Autodesk Inventor part; units mm, degrees
ref_plane "Start plane" through (0, 0, 0) normal (0, 0, 1) x (1, 0, 0)
ref_plane "End plane" through (0, 0, 609.6) normal (0, 0, 1) x (1, 0, 0)
ref_plane "YZ Plane" through (0, 0, 0) normal (1, 0, 0) x (0, 1, 0)
ref_plane "Start plane" through (0, 0, 0) normal (0, 0, 1) x (1, 0, 0)
ref_plane "End plane" through (0, 0, 609.6) normal (0, 0, 1) x (1, 0, 0)
sketch "Sketch" plane through (0, 0, 0) normal (0, 0, 1) x (1, 0, 0)
  line L0 (-25.4, -12.7) -> (-25.4, 12.7)
  line L1 (-12.7, 25.4) -> (12.7, 25.4)
  line L2 (25.4, 12.7) -> (25.4, -12.7)
  line L3 (12.7, -25.4) -> (-12.7, -25.4)
  arc A0 (-25.4, -12.7) -> (-12.7, -25.4) centre (-12.7, -12.7) ccw
  arc A1 (-12.7, 25.4) -> (-25.4, 12.7) centre (-12.7, 12.7) ccw
  arc A2 (25.4, 12.7) -> (12.7, 25.4) centre (12.7, 12.7) ccw
  arc A3 (12.7, -25.4) -> (25.4, -12.7) centre (12.7, -12.7) ccw
  arc A4 (-12.7, 19.05) -> (-19.05, 12.7) centre (-12.7, 12.7) ccw
  line L4 (-12.7, 19.05) -> (12.7, 19.05)
  arc A5 (19.05, 12.7) -> (12.7, 19.05) centre (12.7, 12.7) ccw
  line L5 (19.05, 12.7) -> (19.05, -12.7)
  arc A6 (12.7, -19.05) -> (19.05, -12.7) centre (12.7, -12.7) ccw
  line L6 (12.7, -19.05) -> (-12.7, -19.05)
  arc A7 (-19.05, -12.7) -> (-12.7, -19.05) centre (-12.7, -12.7) ccw
  line L7 (-19.05, -12.7) -> (-19.05, 12.7)
  line L8 (0, 39.2424) -> (0, -39.2424) construction
  line L9 (-39.2424, 0) -> (39.2424, 0) construction
  dimension "d10" = 50.8
  dimension "d11" = 50.8
  dimension "d12" = 6.35
  dimension "d15" = 25.4
  dimension "d16" = 25.4
  dimension "d17" = 12.7
extrude "Body" add sketch "Sketch" along normal up to surface (609.6 mm away) from surface at 0
sketch "Sketch3" plane through (0, 0, 0) normal (0, 0, 1) x (1, 0, 0)
  line L0 (0, 0) -> (10, 0)
ref_plane "Work Plane3" through (0, 0, 0) normal (0, -1, 0) x (1, 0, 0)
sketch "Sketch4" plane through (0, 0, 0) normal (0, -1, 0) x (1, 0, 0)
  line L0 (-2, 0) -> (12, 0)
  line L1 (-2, 609.6) -> (12, 609.6)
  dimension "d19" = 609.6
sketch "Sketch5" plane through (25.4, -12.7, 609.6) normal (1, 0, 0) x (0, 0, -1)
  line L0 (609.6, 25.4) -> (609.6, 38.1)
  line L1 (609.6, 25.4) -> (609.6, 0)
  line L2 (609.6, -12.7) -> (609.6, 0)
  line L3 (609.6, 38.1) -> (606.895, 38.1)
  line L4 (606.895, 38.1) -> (609.5275, 8.0103)
  line L5 (609.6, -12.7) -> (590.55, -12.7)
  arc A0 (609.6, 6.35) -> (609.5275, 8.0103) centre (590.55, 6.35) ccw
  arc A1 (590.55, -12.7) -> (609.6, 6.35) centre (590.55, 6.35) ccw
  line L6 (0, 25.4) -> (0, 38.1)
  line L7 (0, 25.4) -> (0, 0)
  line L8 (0, -12.7) -> (0, 0)
  line L9 (0, -12.7) -> (4.4444, -12.7)
  line L10 (4.4444, -12.7) -> (0, 38.1)
  point P0 (609.6, 12.7)
  dimension "d20" = 5
  dimension "d23" = 19.05
extrude "Extrusion2" cut sketch "Sketch5" against normal through all
hole "Hole1" at (25.4, -6.35, 19.05) direction (-1, 0, 0) diameter 12.7 end through all
sketch "Sketch6" plane through (25.4, 12.7, 608.4889) normal (1, 0, 0) x (0, 0, -1)
  point P0 (608.4889, -12.7)
  point P1 (557.6889, -6.35)
  dimension "d33" = 50.8
  dimension "d34" = 6.35
hole "Hole2" at (25.4, 6.35, 50.8) direction (-1, 0, 0) diameter 12.7 end through all
equation "\"d10\" = G_H"
equation "\"d11\" = G_W"
equation "\"d12\" = G_T"
equation "\"d15\" = 0.5 * d10"
equation "\"d16\" = 0.5 * d11"
equation "\"d17\" = G_IR"
equation "\"d3\" = G_L"
equation "\"G_W\" = 50.8"
equation "\"G_H\" = 50.8"
equation "\"G_T\" = 6.35"
equation "\"G_IR\" = 12.7"
equation "\"G_L\" = d19"
equation "\"G_OFFSET_START\" = 0"
equation "\"G_OFFSET_END\" = 0"
equation "\"d14\" = G_OFFSET_END + B_L"
equation "\"B_L\" = 609.6"
properties part number "A1-18002-200-01 Leg tube" material "Steel, Mild"
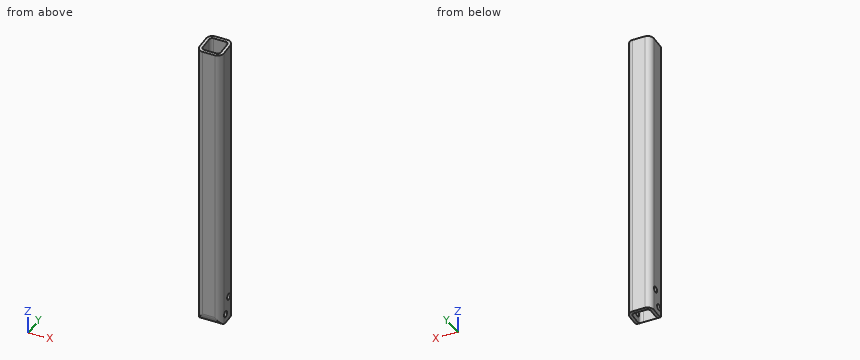
Here's how the part is built. I have some questions about the finished solid (model axes, mm). Round coordinates to 2 decimals unless told otherwise and drop trailing zeros. Order: outer loops, then holes, each group sorted by start corner. A loop starts at its lowest first (then second) coordinate and runs counter-clockwise, first axis right, second up. Notation, with made-up numbers: (-9, 36.5) -> (5, 36.5) arc R24 ccw to (5, 64.5) -> close; hole circle Ø2 at (-15, -8). An arc over 180 degrees is marked (long way). Use a Markdown table: item, result. Add a question column.
(1) For pin 1 Ø3 at (x, z) = (18.5, 372.5) entering from -Y; pin 2 Ø3 at (y, z) = (-15.5, 126.5) entering from -X; pin 3 Ø6 at (y, z) = (19.5, 418.5) entering from -X, each with a flat end and sliding along its axis, tell me the tip position at first contact or that it passes through.
(2) Suppose I cut it at C-C, the plane y = 6.35. Please give me the cut outline in (x, z).
(3) Suppose I cut it at B-B, the plane z = 169. Please give me the cut outline in (x, y), and give its area (3 significant figures).
(4) I need wall thicknesses on line 1 along X through (y, z) = (10, 542.5); line 2 along Y through (x, z) = (-22.25, 19.05). Which ranges of each line are inside material? Lowest first, please.
(5) Suppose I cut it at A-A, the plane x = 3.5. Please give me the cut outline in (y, z) (3 decimals).
Verdict:
| question | item | result |
|---|---|---|
| 1 | pin 1 | y = -24.65 |
| 1 | pin 2 | x = -25.33 |
| 1 | pin 3 | x = -24.82 |
| 2 | outline | (-25.4, 1.04) -> (-19.05, 1.04) -> (-19.05, 44.45) -> (-25.4, 44.45) -> close; (-25.4, 57.15) -> (-19.05, 57.15) -> (-19.05, 607.93) -> (-25.4, 607.93) -> close; (19.05, 1.04) -> (25.4, 1.04) -> (25.4, 44.45) -> (19.05, 44.45) -> close; (19.05, 57.15) -> (25.4, 57.15) -> (25.4, 607.93) -> (19.05, 607.93) -> close |
| 3 | outline | (-25.4, -12.7) arc R12.7 ccw to (-12.7, -25.4) -> (12.7, -25.4) arc R12.7 ccw to (25.4, -12.7) -> (25.4, 12.7) arc R12.7 ccw to (12.7, 25.4) -> (-12.7, 25.4) arc R12.7 ccw to (-25.4, 12.7) -> close; hole (-19.05, -12.7) arc R6.35 ccw to (-12.7, -19.05) -> (12.7, -19.05) arc R6.35 ccw to (19.05, -12.7) -> (19.05, 12.7) arc R6.35 ccw to (12.7, 19.05) -> (-12.7, 19.05) arc R6.35 ccw to (-19.05, 12.7) -> close |
| 3 | area | 1,030 mm2 |
| 4 | line 1 | -25.4 to -19.05, 19.05 to 25.4 |
| 4 | line 2 | -21.07 to -12.7, 0 to 21.07 |
| 5 | outline | (-25.4, 19.05) arc R19.05 ccw to (-19.05, 4.851) -> (-19.05, 605.711) -> (-25.4, 605.156) -> close; (19.05, 2.149) -> (25.4, 2.705) -> (25.4, 609.6) -> (19.05, 609.044) -> close |
